Could you check a few things on this drawing? It's one solid part, dimensions in mm from its lowest x, y, z. Give positions to 0.01 mm unless a question says otherwise; leave off trailing zeros. Loops run counter-clockwise (first coordinate to the right, second up) from the corner with the lowest first, then second, coordinate; pieces in that order, holes last. Notation, with made-up numbers: M 22,-15.75 L 51,-15.75 A22 ccw 51,20.25 Z; hole C 54.5,-7 d11. An arc over 180 degrees is marked long. Answer as a JSON object with one key per item and string values.
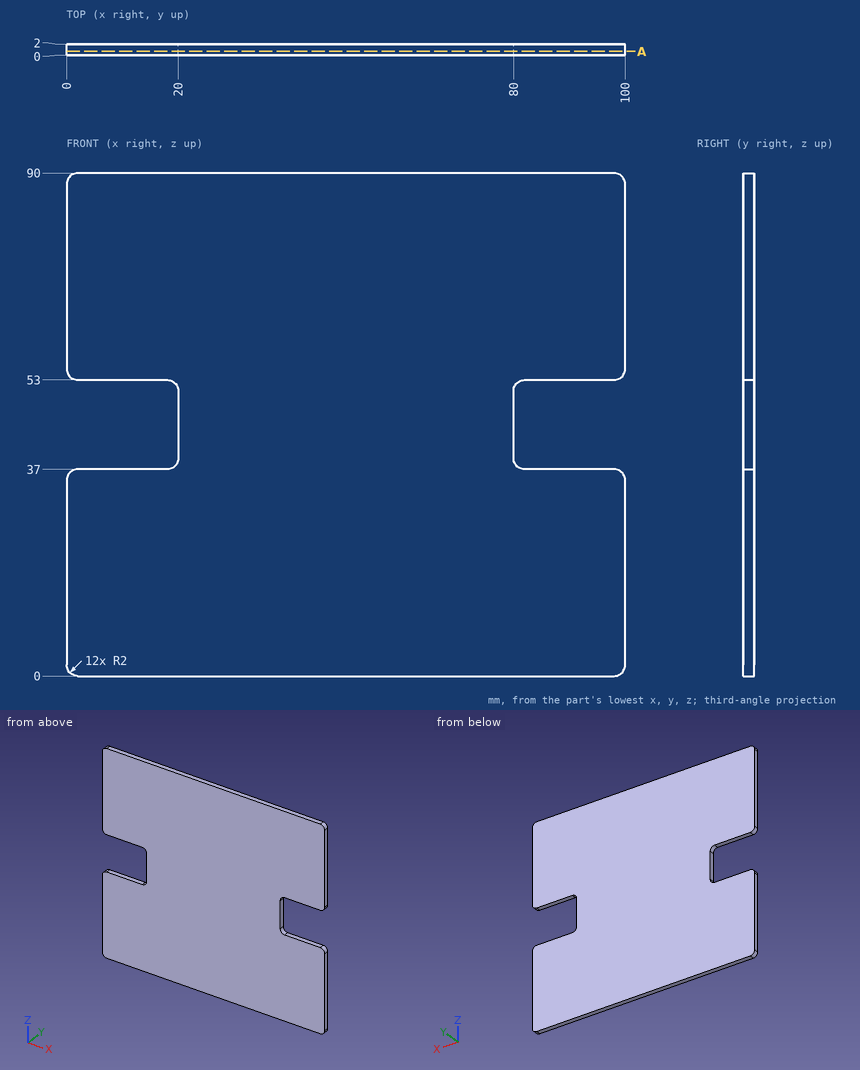
1) Suppose I cut it at A-A, the plane y = 0.7. Write out the boundary of the cut face in (x, z).
Answer list:
{"outline": "M 0,2 A2 ccw 2,0 L 98,0 A2 ccw 100,2 L 100,35 A2 ccw 98,37 L 82,37 A2 cw 80,39 L 80,51 A2 cw 82,53 L 98,53 A2 ccw 100,55 L 100,88 A2 ccw 98,90 L 2,90 A2 ccw 0,88 L 0,55 A2 ccw 2,53 L 18,53 A2 cw 20,51 L 20,39 A2 cw 18,37 L 2,37 A2 ccw 0,35 Z"}
2) Please list where these lines run through material, in increasing order: line 1 along Z through (x, y) = (94.5, 1.2); line 2 along X through (y, z) = (1.5, 46). Write a range as from..to.
Answer list:
{"line 1": "0..37, 53..90", "line 2": "20..80"}
3) Will these pins go through, and if not, where does the flat tip stop? pin 1 Ø1 at (y, z) = (1.5, 38) entering from -X; pin 2 Ø1 at (y, z) = (0.5, 42.5) entering from -X.
Answer list:
{"pin 1": "x = 19.32", "pin 2": "x = 20"}
